Verification items for the finished model (mm, model axes). Give positions to 0.01 mm unless a question says otherwise; leave off trailing zeros. Use a Markdown table: item, result.
from build123d import *

# Parameters (mm, degrees)
F0_W             = 20
F0_H             = 20
F1_DEPTH         = 413
F2_R             = 2.1
F3_DEPTH         = 413.001
F4_R             = 1
F6_DEPTH         = 413.001
F6_COPIES3_COUNT = 2
F6_COPIES3_ANGLE = 90
F6_COPIES4_COUNT = 2
F6_COPIES4_ANGLE = 270
F6_COPIES6_COUNT = 2
F9_W             = 16.4
F9_H             = 6.8613203436
F10_DEPTH        = 413.001
F12_DEPTH        = 413


# Not quite as in the source:
# - a pattern or mirror of a feature is missing from the dataset's text; its kind, count and spacing are read off the source's solid


with BuildPart() as f1:
    # F0 (on Front) → F1 (new body)
    with BuildSketch(Plane.XZ):
        Rectangle(F0_W, F0_H)
    extrude(amount=F1_DEPTH)

    # F2 (on face) → F3 (cut, through all)
    with BuildSketch(Plane.XZ.offset(413)):
        Circle(F2_R)
    extrude(amount=-F3_DEPTH, mode=Mode.SUBTRACT)

    # F4
    f4_edges = [f1.edges().sort_by_distance(p)[0] for p in [
        (-10, -206.5, 10),
        (10, -206.5, 10),
    ]]
    fillet(f4_edges, radius=F4_R)

    # F5 (on face) → F6 (cut, through all)
    with BuildSketch(Plane.XZ.offset(413)):
        Polygon((0, 3.9006601718), (0, 10), (-2.84, 10), (-4.64, 10), (-2.84, 8.2), (-5.4993398282, 8.2), (-5.4993398282, 6.56), (-2.84, 3.9006601718), align=None)
        Polygon((-6.5693398282, 8.2), (-8.2, 8.2), (-7.0953059148, 7.0953059148), (-6.5693398282, 7.6212720014), align=None)
    f6 = extrude(amount=-F6_DEPTH, mode=Mode.SUBTRACT)

    # F6_copies: F6 across plane
    add(f6.mirror(Plane(origin=(0, 0, 0), x_dir=(-0.7071067812, 0, -0.7071067812), z_dir=(0.7071067812, 0, -0.7071067812))), mode=Mode.SUBTRACT)

    # F6_copies1: F6 across plane
    add(f6.mirror(Plane(origin=(0, 0, 0), x_dir=(0.7071067812, 0, -0.7071067812), z_dir=(-0.7071067812, 0, -0.7071067812))), mode=Mode.SUBTRACT)

    # F6_copies2: F6 across plane
    add(f6.mirror(Plane(origin=(0, 0, 0), x_dir=(0, 0, 1), z_dir=(1, 0, 0))), mode=Mode.SUBTRACT)

    # F6_copies3: F6 ×2 about axis
    f6_copies3_axis = Axis((0, 0, 0), (0, 1, 0))
    for i in range(1, F6_COPIES3_COUNT):
        add(f6.rotate(f6_copies3_axis, i * F6_COPIES3_ANGLE / (F6_COPIES3_COUNT - 1)), mode=Mode.SUBTRACT)

    # F6_copies4: F6 ×2 about axis
    f6_copies4_axis = Axis((0, 0, 0), (0, 1, 0))
    for i in range(1, F6_COPIES4_COUNT):
        add(f6.rotate(f6_copies4_axis, i * F6_COPIES4_ANGLE / (F6_COPIES4_COUNT - 1)), mode=Mode.SUBTRACT)

    # F6_copies5: F6 across plane
    add(f6.mirror(Plane(origin=(0, 0, 0), x_dir=(-1, 0, 0), z_dir=(0, 0, -1))), mode=Mode.SUBTRACT)

    # F6_copies6: F6 ×2 about axis
    f6_copies6_axis = Axis((0, 0, 0), (0, 1, 0))
    for i in range(1, F6_COPIES6_COUNT):
        add(f6.rotate(f6_copies6_axis, i * 360 / F6_COPIES6_COUNT), mode=Mode.SUBTRACT)

    # F8: F1 across face


with BuildPart() as f1_1:
    add(f1.part)
    add(f1.part.mirror(Plane(origin=(-7.32, -206.5, -10), x_dir=(1, 0, 0), z_dir=(0, 0, -1))))

    # F9 (on face) → F10 (cut, through all)
    with BuildSketch(Plane.XZ.offset(413)):
        with Locations((0, -10)):
            Rectangle(F9_W, F9_H)
    extrude(amount=-F10_DEPTH, mode=Mode.SUBTRACT)

    # F11 (on face) → F12 (join, through all)
    with BuildSketch(Plane.XZ.offset(413)):
        with BuildLine():
            ThreePointArc((-9, -10), (-9.7071067812, -9.7071067812), (-10, -9))
            Line((-10, -9), (-10, -11))
            ThreePointArc((-10, -11), (-9.7071067812, -10.2928932188), (-9, -10))
        make_face()
        with BuildLine():
            ThreePointArc((10, -9), (9.7071067812, -9.7071067812), (9, -10))
            ThreePointArc((9, -10), (9.7071067812, -10.2928932188), (10, -11))
            Line((10, -11), (10, -9))
        make_face()
        Polygon((5.9386796564, -6.9993398282), (8.2, -6.9993398282), (8.2, -6.5693398282), (5.5086796564, -6.5693398282), align=None)
        Polygon((-8.2, -6.5693398282), (-8.2, -6.9993398282), (-5.9386796564, -6.9993398282), (-5.5086796564, -6.5693398282), align=None)
    extrude(amount=-F12_DEPTH)


solid = f1_1.part
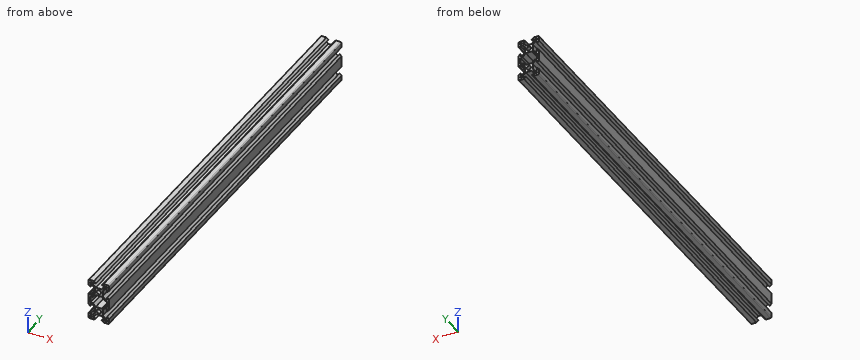
(1) Material ranges on line 1 (Z direction, x = 6.5, y = -43); line 2 (Z direction, x = 0, y = -132.5); line 3 (Z direction, x = -8.5, y = -331), recorded low to high.
Results below:
| item | result |
|---|---|
| line 1 | -30 to -25.44, -14.56 to -13.43, -7 to -5.44, 5.44 to 10 |
| line 2 | -23.9 to -22.1, -17.9 to -16.1, -3.9 to -2.1, 2.1 to 3.9 |
| line 3 | -30 to -23.14, -16.86 to -3.14, 3.14 to 10 |
(2) Gauge pin test, flat ends, axial feed: P1, Ø2, axis at y = -235.5, z = -18.5, coming from the -X side; P2, Ø3, axis at y = -262, z = -24.5, coming from the +X side; P3, Ø2, axis at y = -173.5, z = -3.5, coming from the +X side. Record the tip position at first contact, or that the pin passes through.
Results below:
| item | result |
|---|---|
| P1 | x = -3.9 |
| P2 | x = 10 |
| P3 | x = 9.86 |
(3) Cross-section at A-A on y = -84.5. State how many separate pieces and enclosed holes the cut face has, then the cut area to 3 significant figures.
Results below:
| item | result |
|---|---|
| separate pieces | 1 |
| enclosed holes | 7 |
| area | 286 mm^2 |
